Autodesk Inventor part; units mm, degrees
ref_plane "YZ Plane" through (0, 0, 0) normal (1, 0, 0) x (0, 1, 0)
ref_plane "XZ Plane" through (0, 0, 0) normal (0, 1, 0) x (-1, 0, 0)
ref_plane "XY Plane" through (0, 0, 0) normal (0, 0, 1) x (1, 0, 0)
sketch "Sketch1" plane through (0, 0, 0) normal (1, 0, 0) x (0, 1, 0)
  circle A0 centre (0, 0) radius 4.7625
  dimension "d0" = 9.525
extrude "Extrusion1" add sketch "Sketch1" along normal blind 31.5379
sketch "Sketch2" plane through (31.5379, 0, 0) normal (1, 0, 0) x (0, 0, -1)
  point P0 (0, 0)
  point P1 (0, 0)
hole "Hole1" at (31.5379, 0, 0) direction (-1, 0, 0) diameter 3.9624 depth 13.6144 tip angle 118
sketch "Sketch3" plane through (0, 0, 0) normal (-1, 0, 0) x (0, 0, 1)
  point P0 (0, 0)
  point P1 (0, 0)
hole "Hole2" at (0, 0, 0) direction (1, 0, 0) diameter 3.9624 depth 13.6144 tip angle 118
properties part number "STOCK,REVERSER,STANDOFF" material "Aluminum 6061"
Can you work these out from the model? Positions are in its coordinate system, mm. A direction names the side the tool comes from. Give positions to 0.01 mm unless a question says otherwise; leave off trailing zeros. Order: outer loops, then holes, each group sorted by start corner. A loop starts at its lowest first (then second) coordinate and runs counter-clockwise, first axis right, second up. Notation, with made-up numbers: M 1.5,51.25 L 32.5,51.25 A20 ccw 32.5,66.25 Z; hole C 31.25,59 d1. An arc over 180 degrees is marked long. One line per item, written item: value.
Item 1: If we mould it in two halves opening along Z, with no side actions, what happens to faces 1 (the face through (0, 2, -1)), 2 (the face through (14.598, -0.336, -0.075)), 3 (the face through (15.55, -3.78, 2.9)), 4 (the face through (16.94, -0.34, 0.07))? For each: pulls with the +Z half, pulls with the -Z half, needs draft (parallel to the pull), parting line crosses it, or undercut.
Verdict:
face 1: needs draft
face 2: undercut
face 3: parting line crosses it
face 4: undercut
Item 2: Please list where these lines run through material, in increasing order: line 1 (Z direction, x = 21.5, y = 0); line 2 (Z direction, x = 8, y = -0.75); line 3 (Y direction, x = 6.5, z = -1.5).
Verdict:
line 1: -4.76 to -1.98, 1.98 to 4.76
line 2: -4.7 to -1.83, 1.83 to 4.7
line 3: -4.52 to -1.29, 1.29 to 4.52
Item 3: For pin 1 (2.5 mm diameter, centred on y = 0, z = 0, fed in from -X); pin 2 (1.5 mm diameter, centred on y = 0.5, z = -0.5, fed in from -X), each with a flat end and sliding along its axis, tell me the tip position at first contact or that it passes through.
Verdict:
pin 1: x = 14.05
pin 2: x = 13.93
Item 4: If we section it at C-C on y = -3.5: Write out the boundary of the cut face in (x, z).
Verdict:
outline: M 0,-3.23 L 31.54,-3.23 L 31.54,3.23 L 0,3.23 Z
Item 5: If we section it at B-B on z = 2.5: Write out the boundary of the cut face in (x, y), and give its area (3 significant figures).
Verdict:
outline: M 0,-4.05 L 31.54,-4.05 L 31.54,4.05 L 0,4.05 Z
area: 256 mm2
Item 6: If we section it at D-D on x = 14.5: Write out the boundary of the cut face in (y, z) (1 decimal).
Verdict:
outline: C 0,0 d9.5; hole C 0,0 d1
Item 7: If we section it at A-A on x = 5.5: Write out the boundary of the cut face in (y, z) (1 decimal).
Verdict:
outline: C 0,0 d9.5; hole C 0,0 d4
Item 8: For faces 5 (the face through (6.903, -1.964, -0.258)), 6 (the face through (31.538, 2, -1)), 7 (the face through (24.635, -1.964, 0.258)), which set-ups out of +Z, -Z, +X, -X, +Y, -Y let a thin tool reach every point of the face, with its end or its side?
Verdict:
face 5: -X
face 6: +Z, -Z, +X, +Y, -Y
face 7: +X
